Autodesk Inventor part; units mm, degrees
ref_plane "YZ Plane" through (0, 0, 0) normal (1, 0, 0) x (0, 1, 0)
ref_plane "XZ Plane" through (0, 0, 0) normal (0, 1, 0) x (-1, 0, 0)
ref_plane "XY Plane" through (0, 0, 0) normal (0, 0, 1) x (1, 0, 0)
sketch "Náčrt1" plane through (0, 0, 0) normal (0, 1, 0) x (-1, 0, 0)
  line L0 (20, 0) -> (40, 0)
  line L1 (40, 0) -> (40, -40)
  line L2 (40, -40) -> (36, -40)
  line L3 (36, -40) -> (36, -46)
  circle A0 centre (50, -53) radius 3.5
  arc A1 (55.6, -57.2) -> (50, -46) centre (50, -53) ccw
  line L4 (36, -46) -> (50, -46)
  arc A2 (20, -96.5) -> (20, -89.5) centre (20, -93) ccw
  arc A3 (20, -100) -> (25.6, -97.2) centre (20, -93) ccw
  line L5 (55.6, -57.2) -> (25.6, -97.2)
  line L6 (20, 0) -> (0, 0)
  line L7 (0, 0) -> (0, -40)
  line L8 (0, -40) -> (4, -40)
  line L9 (4, -40) -> (4, -46)
  circle A4 centre (-10, -53) radius 3.5
  arc A5 (-10, -46) -> (-15.6, -57.2) centre (-10, -53) ccw
  line L10 (4, -46) -> (-10, -46)
  arc A6 (20, -89.5) -> (20, -96.5) centre (20, -93) ccw
  arc A7 (14.4, -97.2) -> (20, -100) centre (20, -93) ccw
  line L11 (-15.6, -57.2) -> (14.4, -97.2)
  dimension "d0" = 40
  dimension "d1" = 40
  dimension "d2" = 4
  dimension "d3" = 6
  dimension "d8" = 7
  dimension "d9" = 14
  dimension "d11" = 7
  dimension "d12" = 14
  dimension "d13" = 60
extrude "Deska1" add sketch "Náčrt1" along normal blind 2
sketch "Náčrt2" plane through (-38, 0, 0) normal (-1, 0, 0) x (0, -1, 0)
  line L0 (0, -40) -> (0, 0)
  line L1 (0, 0) -> (-15, 0)
  line L2 (-15, 0) -> (-15, -40)
  line L3 (-15, -40) -> (0, -40)
edge flange "Obruba1" height 15 angle 90 thickness 2 bend radius 2 thickness toward (-1, 0, 0) relief tear relief width 2 relief depth 1 corner gap 2 corner form 0 edges at (-40, 2, -20) (0, 2, -20) wall of the first edge with corners at (-38, 0, -40) (-38, 0, 0) (-38, 15, 0) (-38, 15, -40)
bend "Ohyb1"
corner "Roh1"
chamfer "Zkosení rohu1" distance 3 angle 45 4 edges at (-39, 15, -40) (-39, 15, 0) (-1, 15, -40) (-1, 15, 0)
sketch "Náčrt3" plane through (0, 2, 0) normal (0, 1, 0) x (1, 0, 0)
  line L0 (-4, 0) -> (-36, 0) construction
  line L1 (-40, 40) -> (-40, 0) construction
  point P0 (0, 0)
  point P1 (-20, 20)
  dimension "d28" = 20
  dimension "d29" = 20
hole "Díra1" at (-20, 2, -20) direction (0, -1, 0) diameter 16 depth 2 tip angle 118
sketch "Náčrt5" plane through (0, 2, 0) normal (0, 1, 0) x (1, 0, 0)
  line L0 (-4, 0) -> (-36, 0) construction
  line L1 (-40, 37) -> (-40, 3) construction
  point P0 (0, 0)
  point P1 (-20, 60)
  dimension "d46" = 60
  dimension "d47" = 20
hole "Díra3" at (-20, 2, -60) direction (0, -1, 0) diameter 16 depth 2 tip angle 118
equation "\"d35\" = Tloušťka"
equation "\"d53\" = Tloušťka"
equation "\"d14\" = Tloušťka"
equation "\"d15\" = ŠířkaVýštipu"
equation "\"d16\" = HloubkaVýštipu"
equation "\"d17\" = MinimálníZbytek"
equation "\"d18\" = PřechodovýPoloměr"
equation "\"d21\" = PoloměrOhybu"
equation "\"d22\" = VelikostRohovéhoVýštipu"
equation "\"d23\" = VelikostMezery"
equation "\"d24\" = VelikostJacobihoPoloměru"
equation "\"PoloměrOhybu\" = Tloušťka"
equation "\"ŠířkaVýštipu\" = Tloušťka"
equation "\"HloubkaVýštipu\" = 0.5 * Tloušťka"
equation "\"VelikostRohovéhoVýštipu\" = 4 * Tloušťka"
equation "\"MinimálníZbytek\" = 2 * Tloušťka"
equation "\"PřechodovýPoloměr\" = PoloměrOhybu"
equation "\"VelikostJacobihoPoloměru\" = PoloměrOhybu"
equation "\"VelikostMezery\" = Tloušťka"
properties part number "26886-Vodička_Vojtěch_příklad-4"
For this review, take the finished solid that the model builds, in its own axes (mm). A direction names the side the tool comes from. Give positions to 0.01 mm unless a question says otherwise; leave off trailing zeros. Order: outer loops, then holes, each group sorted by start corner. A loop starts at its lowest first (then second) coordinate and runs counter-clockwise, first axis right, second up.
1) Take a section at B-B (z = -93). Give the boundary of the cut face in (x, y), then the cut area to 3 significant figures.
2) Take a section at D-D (z = -20). Give the boundary of the cut face in (x, y).
3) Wall thickness on line 1 (X direction, y = 9.75, z = -37); line 2 (Y direction, x = -17, z = -78); line 3 (Z direction, x = -50, y = 0.5): over which ranges is each line inside the solid? List them lowest first.
4) Take a section at A-A (x = -20). Give the boundary of the cut face in (y, z), then the cut area to 3 significant figures.
5) Take a section at C-C (y = 8.25). Give the boundary of the cut face in (x, z).
6) The part is to be moulded in two halves that separate along Z. For faces 4 (the face through (-1, 14, -2)), 5 (the face through (-4, 1, -43)), 6 (the face through (-2, 9, -20)), say which applies: released by +Z, released by -Z, zero draft, split by the parting line, or undercut.
7) For faces 1 (the face through (-37.43, 2.6, -19.72)), 2 (the face through (-36, 1, -43)), 3 (the face through (-1.141, 1.203, -20.28)), list the 3-axis set-ups (+Z, -Z, +X, -X, +Y, -Y) from which the entire face can be reached by the end or side of a thin tool; tool diameter is ignored.
8) Insertion check: pin 1 (18.5 mm diameter, centred on x = -20, z = -20, fed in from -Y); pin 2 (3.5 mm diameter, centred on y = 7.5, z = -14.5, fed in from +X); pin 3 (1.6 mm diameter, centred on y = 0.5, z = -42, fed in from -X); pin 4 (1 mm diameter, centred on x = -45.5, y = 1, fed in from +Z). Each pin has a flat end and moves straight along its axis. Give the tip position at first contact, or say it passes through.
Derived:
1. outline: (-28.75, 0) - (-23.5, 0) - (-23.5, 2) - (-28.75, 2) - close; (-16.5, 0) - (-11.25, 0) - (-11.25, 2) - (-16.5, 2) - close
1. area: 21.0 mm2
2. outline: (-40, 4) arc R4 ccw to (-36, 0) - (-28, 0) - (-28, 2) - (-36, 2) arc R2 cw to (-38, 4) - (-38, 15) - (-40, 15) - close; (-12, 0) - (-4, 0) arc R4 ccw to (0, 4) - (0, 15) - (-2, 15) - (-2, 4) arc R2 cw to (-4, 2) - (-12, 2) - close
3. line 1: x = -40 to -38, -2 to 0
3. line 2: y = 0 to 2
3. line 3: z = -64.67 to -56.5, -49.5 to -46
4. outline: (0, -100) - (2, -100) - (2, -96.5) - (0, -96.5) - close; (0, -89.5) - (2, -89.5) - (2, -68) - (0, -68) - close; (0, -52) - (2, -52) - (2, -28) - (0, -28) - close; (0, -12) - (2, -12) - (2, 0) - (0, 0) - close
4. area: 122 mm2
5. outline: (-40, -40) - (-38, -40) - (-38, 0) - (-40, 0) - close; (-2, -40) - (0, -40) - (0, 0) - (-2, 0) - close
6. face 4: released by +Z
6. face 5: undercut
6. face 6: zero draft
7. face 1: +Z, -Z, +Y
7. face 2: -X, +Y, -Y
7. face 3: +Z, +X, -Y
8. pin 1: stops at y = 0
8. pin 2: stops at x = 0
8. pin 3: stops at x = -36
8. pin 4: stops at z = -46
